Here's how the part is built. I have some questions about the finished solid (model axes, mm). A direction names the side the tool comes from. Give positions to 0.01 mm unless a question says otherwise; leave off trailing zeros. Write each loop counter-clockwise with the first axis right and the second up, starting at its lowest first coordinate (ties: lowest second). Pieces come first, ordered by that corner, then holes. Notation, with made-up numbers: (75, 7) - (82, 7) arc R14 ccw to (82, 18) - close; hole circle Ø2 at (-36, 63.25). An arc over 180 degrees is marked (long way). Use a Markdown table: item, result.
```python
from build123d import *

# Parameters (mm, degrees)
CHANFREIN2_SIZE = 1
M_PLATS_DEPTH   = 97.363893653


with BuildPart() as part:
    # Esquisse1 → Forme de révolution (revolve)
    with BuildSketch(Plane.XY, mode=Mode.PRIVATE) as forme_de_r_volution_sk:
        with BuildLine():
            Line((-15, 0), (89.91678311, 0))
            Line((89.91678311, 0), (91.869580122, 3.25))
            Line((91.869580122, 3.25), (92.700961894, 3.25))
            ThreePointArc((92.700961894, 3.25), (94, 3.5), (95.299038106, 3.25))
            Line((95.299038106, 3.25), (97, 3.25))
            Line((97, 3.25), (97.5, 3.75))
            Line((97.5, 3.75), (97.5, 4.92655))
            Line((97.5, 4.92655), (96.42655, 6))
            Line((96.42655, 6), (7.5, 6))
            Line((7.5, 6), (7.5, 4.75))
            Line((7.5, 4.75), (3.5, 4.75))
            Line((3.5, 4.75), (3.5, 15))
            Line((3.5, 15), (0, 15))
            Line((0, 15), (0, 6))
            Line((0, 6), (-15, 6))
            Line((-15, 6), (-15, 0))
        make_face()
    revolve(forme_de_r_volution_sk.sketch.rotate(Axis((110.666531714, 0, 0), (-1, 0, 0)), 90), axis=Axis((110.666531714, 0, 0), (-1, 0, 0)))

    # Chanfrein2
    chanfrein2_edges = [part.edges().sort_by_distance(p)[0] for p in [
        (-15, 0, 6),
    ]]
    chamfer(chanfrein2_edges, length=CHANFREIN2_SIZE)

    # Esquisse3 → Méplats (cut, symmetric)
    with BuildSketch(Plane(origin=(3.5, 0, 0), x_dir=(0, 0, -1), z_dir=(1, 0, 0))):
        Polygon((-103.669154566, 10), (-15.223201291, 10), (13.534968643, 10), (101.980921918, 10), (101.980921918, 186.891906549), (-103.669154566, 186.891906549), align=None)
    m_plats = extrude(amount=M_PLATS_DEPTH, both=True, mode=Mode.SUBTRACT)

    # Symétrie1: Méplats across plane
    add(m_plats.mirror(Plane.ZX), mode=Mode.SUBTRACT)


solid = part.part
```
Item 1: If we section it at C-C, the plane y = 7: Write out the boundary of the cut face in (x, z).
Values:
| item | result |
|---|---|
| outline | (0, -13.27) - (3.5, -13.27) - (3.5, 13.27) - (0, 13.27) - close |
Item 2: If we section it at A-A, the plane x = 29: Write out the boundary of the cut face in (y, z).
Values:
| item | result |
|---|---|
| outline | circle Ø12 at (0, 0) |
Item 3: If we section it at B-B, the plane z = -7.5: Write out the boundary of the cut face in (x, y).
Values:
| item | result |
|---|---|
| outline | (0, -10) - (3.5, -10) - (3.5, 10) - (0, 10) - close |
Item 4: Will these pins go through, and if not, where does the flat tip stop? pin 1 Ø2 at (y, z) = (2.5, -9) entering from +X; pin 2 Ø1 at (x, y) = (84.5, 6) entering from +Z; pin 3 Ø5 at (y, z) = (0, 0) entering from +X.
Values:
| item | result |
|---|---|
| pin 1 | stops at x = 3.5 |
| pin 2 | stops at z = 2.4 |
| pin 3 | stops at x = 91.42 |
Item 5: Thinking about a two-plate mould opening in Z: for faces 1 (the cylindrical face through (92.291, 1.978, 2.579)), 2 (the cylindrical face through (2, 0, 15)), 3 (the cylindrical face through (51.341, -1.802, -5.723)), 4 (the flat face through (2, 10, 0)), which applies, +Z half, -Z half, draft (parallel to the pull), parting line (faces both ways), or undercut?
Values:
| item | result |
|---|---|
| face 1 | undercut |
| face 2 | +Z half |
| face 3 | parting line |
| face 4 | draft |
Item 6: I need wall thicknesses on line 1 along Y through (x, z) = (96.1, 0); line 2 along X through (y, z) = (7.5, 10); line 3 along Y through (x, z) = (96.5, 0). Which ranges of each line are inside material? Lowest first, please. Write a range as [from, to].
Values:
| item | result |
|---|---|
| line 1 | y = [-6, -3.25], [3.25, 6] |
| line 2 | x = [0, 3.5] |
| line 3 | y = [-5.93, -3.25], [3.25, 5.93] |
Item 7: For faces 5 (the cylindrical face through (-7.098, -1.802, -5.723)), 6 (the flat face through (2, -10, 0)), 7 (the cylindrical face through (5.472, 4.637, 1.03)), 8 (the cylindrical face through (96.161, 1.978, 2.579)), 9 (the cylindrical face through (2, 0, -15)), which set-ups out of +Z, -Z, +X, -X, +Y, -Y let a thin tool reach every point of the face, with its end or its side?
Values:
| item | result |
|---|---|
| face 5 | -X |
| face 6 | +Z, -Z, +X, -X, -Y |
| face 7 | none |
| face 8 | +X |
| face 9 | -Z, +X, -X |
